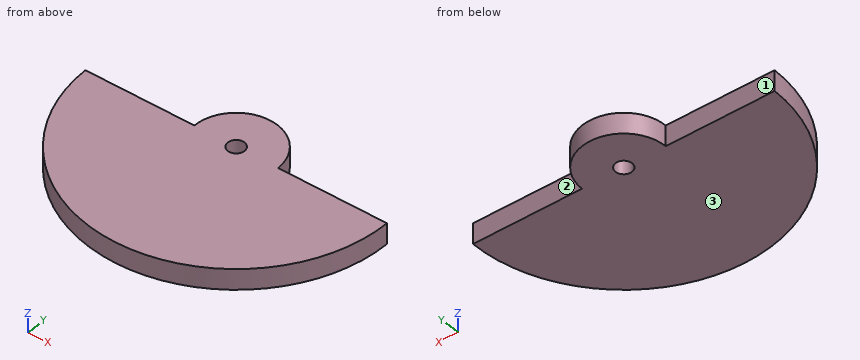
from build123d import *

# Parameters (mm, degrees)
F0_R     = 2
F1_DEPTH = 5


with BuildPart() as f1:
    # F0 (on Top) → F1 (new body)
    with BuildSketch(Plane.XY):
        with BuildLine():
            ThreePointArc((10, 0), (0, 10), (-10, 0))
            Line((-10, 0), (-36, 0))
            ThreePointArc((-36, 0), (0, -36), (36, 0))
            Line((36, 0), (10, 0))
        make_face()
        Circle(F0_R, mode=Mode.SUBTRACT)
    extrude(amount=F1_DEPTH)


solid = f1.part
Design review of the part built by this model. Coordinates are the model's own, in mm. Face numbers are marked on the shaded views. A direction names the side the tool comes from. Round coordinates to 2 decimals unless told otherwise and drop trailing zeros. Write each loop counter-clockwise with the first axis right and the second up, starting at its lowest first coordinate (ties: lowest second). Pieces come first, ordered by that corner, then holes. Notation, with made-up numbers: (-10, -37.5) - (0, -37.5) arc R25 cw to (0, -11.5) - close; hole circle Ø1 at (51.25, 63.5). An arc over 180 degrees is marked (long way). Use a Markdown table: item, result. Add a question column.
1. We need section C-C (z = 3.7). State the section outline as (x, y) points, then the cut area to 3 significant figures.
2. Wall thickness on probe 1 along Y at (x, z) = (0, 2.7); probe 2 along X at (y, z) = (-1.5, 1.6); probe 3 along X at (y, z) = (-33, 2.05): over which ranges is each line inside the solid? List them lowest first.
3. Clearance check with flat-ended pins moving along their axes: pin 1 (2.5 mm diameter, centred on x = -21.5, z = 2.5, fed in from +Y); pin 2 (3 mm diameter, centred on x = 0, y = 0, fed in from +Z); pin 3 (3 mm diameter, centred on y = -4, z = 1.5, fed in from +X); pin 4 (10 mm diameter, centred on x = 24, y = -28.5, fed in from -Z). State where each tip first meets the part, or that it passes through.
4. We need section D-D (x = 32.5). State the section outline as (y, z) points, then the cut area to 3 significant figures.
5. For the marked faces 1, 2 and 3, list the 3-axis set-ups (+Z, -Z, +X, -X, +Y, -Y) from which the entire face can be reached by the end or side of a thin tool; tool diameter is ignored.
6. We need section B-B (y = -1). State the section outline as (x, z) points, then the cut area to 3 significant figures.
7. We need section A-A (x = 0). State the section outline as (y, z) points, then the cut area to 3 significant figures.
Output:
| question | item | result |
|---|---|---|
| 1 | outline | (-36, 0) arc R36 ccw to (36, 0) - (10, 0) arc R10 ccw to (-10, 0) - close; hole circle Ø4 at (0, 0) |
| 1 | area | 2,180 mm2 |
| 2 | probe 1 | y = -36 to -2, 2 to 10 |
| 2 | probe 2 | x = -35.97 to -1.32, 1.32 to 35.97 |
| 2 | probe 3 | x = -14.39 to 14.39 |
| 3 | pin 1 | stops at y = 0 |
| 3 | pin 2 | passes through |
| 3 | pin 3 | stops at x = 35.91 |
| 3 | pin 4 | stops at z = 0 |
| 4 | outline | (-15.48, 0) - (0, 0) - (0, 5) - (-15.48, 5) - close |
| 4 | area | 77.4 mm2 |
| 5 | face 1 | +Z, -Z, -X, +Y |
| 5 | face 2 | +Z, -Z, +X, +Y |
| 5 | face 3 | -Z, +X, -X, +Y, -Y |
| 6 | outline | (-35.99, 0) - (-1.73, 0) - (-1.73, 5) - (-35.99, 5) - close; (1.73, 0) - (35.99, 0) - (35.99, 5) - (1.73, 5) - close |
| 6 | area | 343 mm2 |
| 7 | outline | (-36, 0) - (-2, 0) - (-2, 5) - (-36, 5) - close; (2, 0) - (10, 0) - (10, 5) - (2, 5) - close |
| 7 | area | 210 mm2 |
